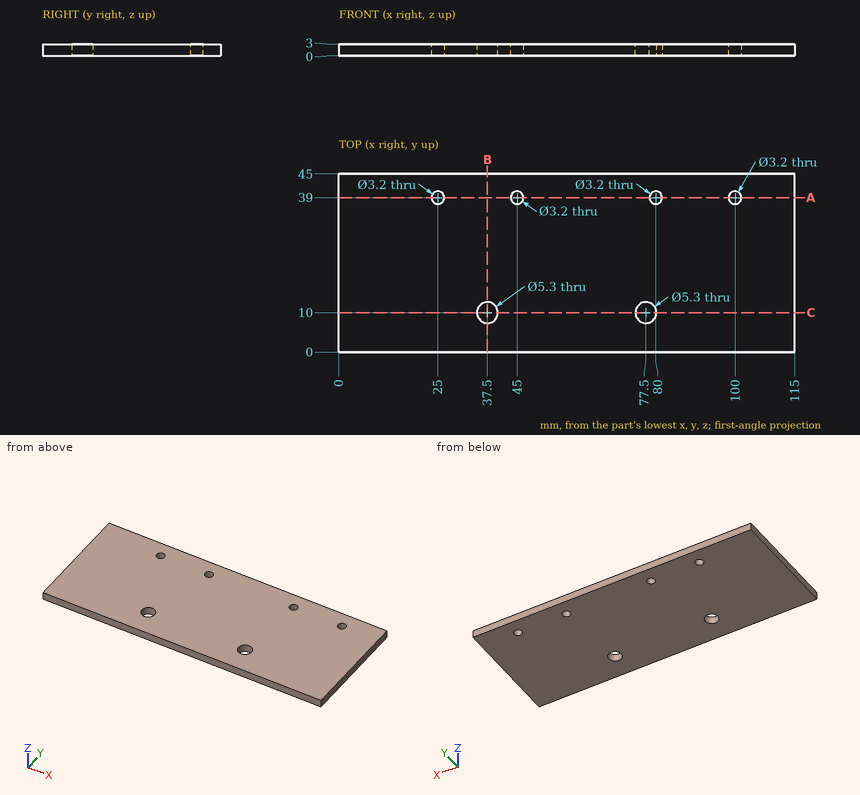
The figure shows three views and two pictorial views of one solid part (mm, origin at its lowest corner). Answer the questions. Coordinates: 2 decimals unless noted, no trailing zeros. Loops run counter-clockwise (first coordinate to the right, second up) from the corner with the lowest first, then second, coordinate; pieces in that order, holes last.
1) Find section C-C on y = 10. Write down the section's boundary in (x, z).
2) Find the intervals of material crossed by L1, parallel to Y at x = 37.5, z = 2.2; L2, parallel to Y at x = 79.5, z = 0.3; L3, parallel to X at y = 9.5, z = 0.7, in increasing order.
3) Find section A-A on y = 39. Write down the section's boundary in (x, z).
4) A flat-ended cylindrical pin translates along its axis: pin 1 Ø8.5 at (x, y) = (77.5, 10) entering from -Z. Find the tip coordinate at first contact, or state that the pin passes through.
5) Find section B-B on x = 37.5. Write down the section's boundary in (y, z).
Values:
1. outline: (0, 0) - (34.85, 0) - (34.85, 3) - (0, 3) - close; (40.15, 0) - (74.85, 0) - (74.85, 3) - (40.15, 3) - close; (80.15, 0) - (115, 0) - (115, 3) - (80.15, 3) - close
2. L1: y = 0 to 7.35, 12.65 to 45
2. L2: y = 0 to 8.26, 11.74 to 37.48, 40.52 to 45
2. L3: x = 0 to 34.9, 40.1 to 74.9, 80.1 to 115
3. outline: (0, 0) - (23.4, 0) - (23.4, 3) - (0, 3) - close; (26.6, 0) - (43.4, 0) - (43.4, 3) - (26.6, 3) - close; (46.6, 0) - (78.4, 0) - (78.4, 3) - (46.6, 3) - close; (81.6, 0) - (98.4, 0) - (98.4, 3) - (81.6, 3) - close; (101.6, 0) - (115, 0) - (115, 3) - (101.6, 3) - close
4. pin 1: stops at z = 0
5. outline: (0, 0) - (7.35, 0) - (7.35, 3) - (0, 3) - close; (12.65, 0) - (45, 0) - (45, 3) - (12.65, 3) - close
